Read the model definition and answer for the solid it produces. Units are mm, in the model's axes. Face numbers are marked on the shaded views. Round coordinates to 2 decimals unless told otherwise and drop trailing zeros. Order: outer loops, then holes, each group sorted by start corner. A loop starts at its lowest first (then second) coordinate and runs counter-clockwise, first axis right, second up. Notation, with made-up numbers: (-33, -27) - (-6, -27) arc R18 cw to (-6, -13) - close; hole circle Ø9 at (-10, 17). An arc over 180 degrees is marked (long way). Answer as a JSON object with one key per item and string values. Group by question number.
Q1. The mould has two halves that part along Y. Classify the marked faces 1, 2, 3 and 4: pulls with the +Y half, pulls with the -Y half, needs draft (parallel to the pull), parting line crosses it, or undercut.
Q2. A cutting plane is placed at D-D on y = -12. Determine the outline of the cut face in (x, z).
Q3. Given pin 1 Ø2 at (x, z) = (-18.5, 8) entering from +Y; pin 2 Ø4 at (x, z) = (-49, 3.5) entering from +Y; pin 3 Ø5 at (x, z) = (-50.5, 5) entering from -Y, each flat-ended and moving along its own axis, determine where each tip first touches the part or whether it passes through.
Q4. A cutting plane is placed at C-C on z = 5.25. Determine the outline of the cut face in (x, y), and give its area (3 significant figures).
Q5. A cutting plane is placed at B-B on y = 0. Determine the outline of the cut face in (x, z), and give its area (3 significant figures).
Q6. Consider line 1 (X direction, y = -0.5, z = 2.5); line 2 (Y direction, x = -50, z = 2.75); line 3 (X direction, y = -16.5, z = 5.5). Determine where each line is inside the solid, lowest interval first.
Q7. A cutting plane is placed at A-A on x = 0. Determine the outline of the cut face in (y, z).
```python
from build123d import *

# Parameters (mm, degrees)
SKETCH1_R           = 26
BOSS_EXTRUDE1_DEPTH = 10
FILLET1_R           = 5
SKETCH2_R           = 4
CUT_EXTRUDE1_DEPTH  = 10


with BuildPart() as part:
    # Sketch1 → Boss-Extrude1 (new body)
    with BuildSketch(Plane.XY):
        with BuildLine():
            Line((31.684802474, 27.352044719), (75.782561157, 27.352044719))
            Line((75.782561157, 27.352044719), (75.782561157, -27.352044719))
            Line((75.782561157, -27.352044719), (31.684802474, -27.352044719))
            ThreePointArc((31.684802474, -27.352044719), (0, -41.857628434), (-31.684802474, -27.352044719))
            Line((-31.684802474, -27.352044719), (-75.782561157, -27.352044719))
            Line((-75.782561157, -27.352044719), (-75.782561157, 27.352044719))
            Line((-75.782561157, 27.352044719), (-31.684802474, 27.352044719))
            ThreePointArc((-31.684802474, 27.352044719), (0, 41.857628434), (31.684802474, 27.352044719))
        make_face()
        Circle(SKETCH1_R, mode=Mode.SUBTRACT)
    extrude(amount=BOSS_EXTRUDE1_DEPTH)

    # Fillet1
    fillet1_edges = [part.edges().sort_by_distance(p)[0] for p in [
        (75.782561157, -27.352044719, 5),
        (31.684802474, -27.352044719, 5),
        (-31.684802474, -27.352044719, 5),
        (-75.782561157, -27.352044719, 5),
        (-75.782561157, 27.352044719, 5),
        (-31.684802474, 27.352044719, 5),
        (31.684802474, 27.352044719, 5),
        (75.782561157, 27.352044719, 5),
    ]]
    fillet(fillet1_edges, radius=FILLET1_R)

    # Sketch2 → Cut-Extrude1 (cut)
    with BuildSketch(Plane.XY.offset(10)):
        with Locations((-50, 0)):
            Circle(SKETCH2_R)
        with Locations((50, 0)):
            Circle(SKETCH2_R)
    extrude(amount=-CUT_EXTRUDE1_DEPTH, mode=Mode.SUBTRACT)


solid = part.part
```
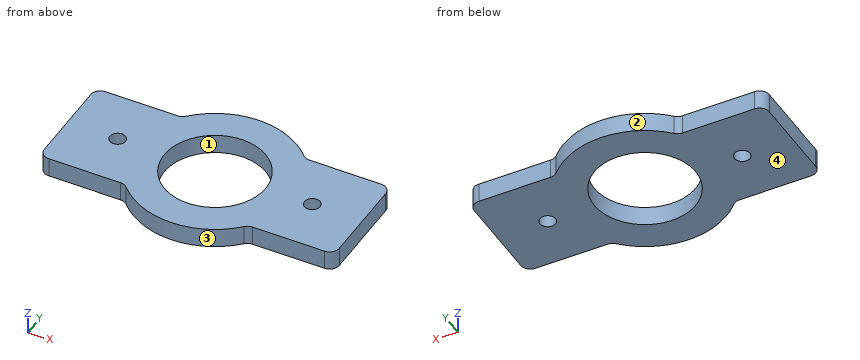
Result set:
{
 "1": {"face 1": "undercut", "face 2": "pulls with the +Y half", "face 3": "pulls with the -Y half", "face 4": "needs draft"},
 "2": {"outline": "(-75.78, 0) - (-23.07, 0) - (-23.07, 10) - (-75.78, 10) - close; (23.07, 0) - (75.78, 0) - (75.78, 10) - (23.07, 10) - close"},
 "3": {"pin 1": "stops at y = 38.02", "pin 2": "stops at y = 27.35", "pin 3": "stops at y = -27.35"},
 "4": {"outline": "(-75.78, -22.35) arc R5 ccw to (-70.78, -27.35) - (-33.9, -27.35) arc R5 cw to (-30.28, -28.9) arc R41.86 ccw to (30.28, -28.9) arc R5 cw to (33.9, -27.35) - (70.78, -27.35) arc R5 ccw to (75.78, -22.35) - (75.78, 22.35) arc R5 ccw to (70.78, 27.35) - (33.9, 27.35) arc R5 cw to (30.28, 28.9) arc R41.86 ccw to (-30.28, 28.9) arc R5 cw to (-33.9, 27.35) - (-70.78, 27.35) arc R5 ccw to (-75.78, 22.35) - close; hole circle Ø8 at (-50, 0); hole circle Ø52 at (0, 0); hole circle Ø8 at (50, 0)", "area": "7,320 mm²"},
 "5": {"outline": "(-75.78, 0) - (-54, 0) - (-54, 10) - (-75.78, 10) - close; (-46, 0) - (-26, 0) - (-26, 10) - (-46, 10) - close; (26, 0) - (46, 0) - (46, 10) - (26, 10) - close; (54, 0) - (75.78, 0) - (75.78, 10) - (54, 10) - close", "area": "836 mm²"},
 "6": {"line 1": "x = -75.78 to -53.97, -46.03 to -26, 26 to 46.03, 53.97 to 75.78", "line 2": "y = -27.35 to -4, 4 to 27.35", "line 3": "x = -75.78 to -20.09, 20.09 to 75.78"},
 "7": {"outline": "(-41.86, 0) - (-26, 0) - (-26, 10) - (-41.86, 10) - close; (26, 0) - (41.86, 0) - (41.86, 10) - (26, 10) - close"}
}
